from build123d import *

# Parameters (mm, degrees)
F0_W     = 1219.2
F0_H     = 1016
F1_DEPTH = 101.6
F2_W     = 1219.2
F2_H     = 127
F3_DEPTH = 152.4


with BuildPart() as f1:
    # F0 (on Top) → F1 (new body)
    with BuildSketch(Plane.XY):
        Rectangle(F0_W, F0_H)
    extrude(amount=F1_DEPTH)

    # F2 (on face) → F3 (join)
    with BuildSketch(Plane(origin=(0, 0, 0), x_dir=(1, 0, 0), z_dir=(0, 0, -1))):
        with Locations((0, 444.5)):
            Rectangle(F2_W, F2_H)
        with Locations((0, -444.5)):
            Rectangle(F2_W, F2_H)
        Rectangle(F2_W, F2_H)
    extrude(amount=F3_DEPTH)


solid = f1.part
Work out the finished part from the listing and answer in its coordinate system (mm). A direction names the side the tool comes from. Give positions to 0.01 mm unless a question says otherwise; leave off trailing zeros. Loops run counter-clockwise (first coordinate to the right, second up) from the corner with the lowest first, then second, coordinate; pieces in that order, holes last. Notation, with made-up numbers: (-14.75, 1.5) -> (44.25, 1.5) arc R4 ccw to (44.25, 8.5) -> close; hole circle Ø6 at (27.25, -25). An arc over 180 degrees is marked (long way). Use a Markdown table: item, result. Add a question column.
1. Find the intervals of material crossed by probe 1 along Y at (x, z) = (396, -48); probe 2 along Z at (x, y) = (-504, 151.5), in increasing order.
2. Section C-C on y = 321.5 is taken. Determine the outline of the cut face in (x, z).
3. Section B-B on x = -44.5 is taken. Determine the outline of the cut face in (y, z), and give its area (3 significant figures).
4. Section A-A on z = -94.5 is taken. Determine the outline of the cut face in (x, y).
5. For faces 1 (the flat face through (-9, -445, -152.4)), 2 (the flat face through (-9, 381, -75)), determine the directions among +Z, -Z, +X, -X, +Y, -Y from which every point of the face is accessible in a straight line to the end or side of a thin tool.
6. A flat-ended cylindrical pin translates along its axis: pin 1 Ø2 at (x, y) = (164.5, 86) entering from -Z. Find the tip coordinate at first contact, or state that the pin passes through.
7. Determine the mould class of faces 3 (the flat face through (-9, 7, 101.6)), 4 (the flat face through (-9, 224, 0)), 5 (the flat face through (-9, -508, -24)), 6 (the flat face through (-9, 508, -27)) for opening direction Y: released by +Y, released by -Y, zero draft, split by the parting line, or undercut.
Results below:
| question | item | result |
|---|---|---|
| 1 | probe 1 | y = -508 to -381, -63.5 to 63.5, 381 to 508 |
| 1 | probe 2 | z = 0 to 101.6 |
| 2 | outline | (-609.6, 0) -> (609.6, 0) -> (609.6, 101.6) -> (-609.6, 101.6) -> close |
| 3 | outline | (-508, -152.4) -> (-381, -152.4) -> (-381, 0) -> (-63.5, 0) -> (-63.5, -152.4) -> (63.5, -152.4) -> (63.5, 0) -> (381, 0) -> (381, -152.4) -> (508, -152.4) -> (508, 101.6) -> (-508, 101.6) -> close |
| 3 | area | 161,000 mm^2 |
| 4 | outline | (-609.6, -508) -> (609.6, -508) -> (609.6, -381) -> (-609.6, -381) -> close; (-609.6, -63.5) -> (609.6, -63.5) -> (609.6, 63.5) -> (-609.6, 63.5) -> close; (-609.6, 381) -> (609.6, 381) -> (609.6, 508) -> (-609.6, 508) -> close |
| 5 | face 1 | -Z, +X, -X, +Y, -Y |
| 5 | face 2 | -Z, +X, -X |
| 6 | pin 1 | stops at z = 0 |
| 7 | face 3 | zero draft |
| 7 | face 4 | undercut |
| 7 | face 5 | released by -Y |
| 7 | face 6 | released by +Y |
